Autodesk Inventor part; units mm, degrees
ref_plane "YZ Plane" through (0, 0, 0) normal (1, 0, 0) x (0, 1, 0)
ref_plane "XZ Plane" through (0, 0, 0) normal (0, 1, 0) x (-1, 0, 0)
ref_plane "XY Plane" through (0, 0, 0) normal (0, 0, 1) x (1, 0, 0)
sketch "Skizze1" plane through (0, 0, 0) normal (0, 0, 1) x (1, 0, 0)
  line L0 (-26, -30) -> (26, -30)
  line L1 (30, -26) -> (30, 26)
  line L2 (26, 30) -> (-26, 30)
  line L3 (-30, 26) -> (-30, -26)
  line L4 (-30, -30) -> (30, 30) construction
  line L5 (30, -30) -> (-30, 30) construction
  arc A0 (30, 26) -> (26, 30) centre (26, 26) ccw
  arc A1 (26, -30) -> (30, -26) centre (26, -26) ccw
  arc A2 (-30, -26) -> (-26, -30) centre (-26, -26) ccw
  arc A3 (-26, 30) -> (-30, 26) centre (-26, 26) ccw
  point P0 (0, 0)
  dimension "d0" = 4
  dimension "d1" = 60
extrude "Extrusion1" add sketch "Skizze1" against normal blind 100
sketch "Skizze2" plane through (0, 0, 0) normal (0, 0, 1) x (1, 0, 0)
  circle A0 centre (0, 0) radius 19.05
  dimension "d4" = 38.1
extrude "Extrusion2" add sketch "Skizze2" along normal blind 1.6
sketch "Skizze4" plane through (0, 0, 0) normal (0, 0, 1) x (1, 0, 0)
  circle A0 centre (0, 0) radius 19.05
  line L0 (30, 26) -> (30, -26)
  arc A1 (30, 26) -> (26, 30) centre (26, 26) ccw
  line L1 (-26, 30) -> (26, 30)
  arc A2 (-26, 30) -> (-30, 26) centre (-26, 26) ccw
  line L2 (-30, -26) -> (-30, 26)
  arc A3 (-30, -26) -> (-26, -30) centre (-26, -26) ccw
  line L3 (26, -30) -> (-26, -30)
  arc A4 (26, -30) -> (30, -26) centre (26, -26) ccw
  line L4 (26, -26) -> (-26, 26) construction
  line L5 (-23.57, 23.57) -> (23.57, 23.57) construction
  line L6 (23.57, 23.57) -> (23.57, -23.57) construction
  line L7 (23.57, -23.57) -> (-23.57, -23.57) construction
  line L8 (-23.57, -23.57) -> (-23.57, 23.57) construction
  line L9 (-23.57, 23.57) -> (23.57, -23.57) construction
  line L10 (23.57, 23.57) -> (-23.57, -23.57) construction
  dimension "d15" = 47.14
hole "Bohrung1" at (23.57, 23.57, 0) at (-23.57, 23.57, 0) at (-23.57, -23.57, 0) at (23.57, -23.57, 0) direction (0, 0, -1) diameter 4.5 end through all
sketch "Skizze5" plane through (0, 0, 1.6) normal (0, 0, 1) x (1, 0, 0)
  circle A0 centre (0, 0) radius 4
  dimension "d23" = 8
extrude "Extrusion4" add sketch "Skizze5" along normal blind 22.4
sketch "Skizze7" plane through (0, 0, -100) normal (0, 0, -1) x (-1, 0, 0)
  circle A0 centre (23.57, -23.57) radius 2.25
  circle A1 centre (-23.57, 23.57) radius 2.25
  circle A2 centre (23.57, 23.57) radius 2.25
  circle A3 centre (-23.57, -23.57) radius 2.25
  line L0 (-30, 26) -> (-30, -26)
  arc A4 (-30, -26) -> (-26, -30) centre (-26, -26) ccw
  line L1 (-26, -30) -> (26, -30)
  arc A5 (26, -30) -> (30, -26) centre (26, -26) ccw
  line L2 (30, -26) -> (30, 26)
  arc A6 (30, 26) -> (26, 30) centre (26, 26) ccw
  line L3 (26, 30) -> (-26, 30)
  arc A7 (-26, 30) -> (-30, 26) centre (-26, 26) ccw
  circle A8 centre (23.57, -23.57) radius 6.43 construction
  line L4 (30, -26) -> (30, 26)
  line L5 (30, -17.14) -> (23.57, -17.14)
  line L6 (-26, -30) -> (26, -30)
  line L7 (17.14, -30) -> (17.14, -23.57)
  arc A9 (23.57, -17.14) -> (17.14, -23.57) centre (23.57, -23.57) ccw
  arc A10 (-17.14, -23.57) -> (-23.57, -17.14) centre (-23.57, -23.57) ccw
  arc A11 (17.2019, 24.4599) -> (23.57, 17.14) centre (23.57, 23.57) ccw
  arc A12 (-23.57, 17.14) -> (-17.14, 23.57) centre (-23.57, 23.57) ccw
  line L8 (23.57, 17.14) -> (30, 17.14)
  line L9 (17.14, 23.57) -> (17.14, 30)
  line L10 (26, 30) -> (-26, 30)
  line L11 (-17.14, 23.57) -> (-17.14, 30)
  line L12 (-23.57, 17.14) -> (-30, 17.14)
  line L13 (-23.57, -17.14) -> (-30, -17.14)
  line L14 (-17.14, -23.57) -> (-17.14, -30)
  point P0 (0, 0)
extrude "Extrusion6" cut sketch "Skizze7" against normal blind 93.2 contours A7 L3 L11 A12 L12 L0 | L13 A10 L14 L1 A4 L0 | L3 A6 L2 L8 A11 L9 | L7 A9 L5 L2 A5 L1
sketch "Skizze8" plane through (0, 0, -100) normal (0, 0, -1) x (-1, 0, 0)
  circle A0 centre (23.57, -23.57) radius 2.25 construction
  circle A1 centre (-23.57, 23.57) radius 2.25 construction
  circle A2 centre (23.57, 23.57) radius 2.25 construction
  circle A3 centre (-23.57, -23.57) radius 2.25 construction
  circle A4 centre (0, 0) radius 19.05 construction
  line L0 (-30, 26) -> (-30, -26) construction
  arc A5 (-26, 30) -> (-30, 26) centre (-26, 26) ccw construction
  line L1 (26, 30) -> (-26, 30) construction
  arc A6 (30, 26) -> (26, 30) centre (26, 26) ccw construction
  line L2 (30, -26) -> (30, 26) construction
  arc A7 (26, -30) -> (30, -26) centre (26, -26) ccw construction
  line L3 (-26, -30) -> (26, -30) construction
  arc A8 (-30, -26) -> (-26, -30) centre (-26, -26) ccw construction
  circle A9 centre (0, 0) radius 42.4264 construction
  line L4 (30, 30) -> (-30, 30) construction
  line L5 (-30, 30) -> (-30, -30) construction
  line L6 (-30, -30) -> (30, -30) construction
  line L7 (30, -30) -> (30, 30) construction
  line L8 (30, 30) -> (-30, -30) construction
  line L9 (-30, 30) -> (30, -30) construction
  line L10 (-17.14, -30) -> (17.14, -30) construction
  line L11 (-30, 17.14) -> (-30, -17.14) construction
equation "\"d1\" = breite"
equation "\"d2\" = Laenge"
equation "\"d4\" = fit"
equation "\"d5\" = fit_l"
equation "\"d15\" = lochabstand"
equation "\"d16\" = bohrung_d"
equation "\"d23\" = schaft_d"
equation "\"d24\" = schaft_l"
equation "\"d28\" = Laenge - Mount_l"
equation "\"breite\" = 60"
equation "\"lochabstand\" = 47.14"
equation "\"schaft_d\" = 8"
equation "\"fit\" = 38.1"
equation "\"fit_l\" = 1.6"
equation "\"Mount_l\" = 6.8"
equation "\"Laenge\" = 100"
equation "\"bohrung_d\" = 4.5"
properties part number "Nema24 - L100" material "Stahl"
Work out the finished part from the listing and answer in its coordinate system (mm). A direction names the side the tool comes from. Coordinates: 2 decimals unless noted, no trailing zeros. Loops run counter-clockwise (first coordinate to the right, second up) from the corner with the lowest first, then second, coordinate; pieces in that order, holes last. Notation, with made-up numbers: M 23,-31.75 L 73,-31.75 A19 ccw 73,-15.75 Z; hole C -7,-7 d9. An arc over 180 degrees is marked long. Use CSV: the item, a comma, the result in double quotes. Start each with the question number.
(1) For faces 4 (the face through (27, 17.14, -54)), 5 (the face through (24, -26, -6.8)), 6 (the face through (-17.14, -27, -54)), 7 (the face through (-0.867, 3.905, 12.643)), determine the directions among +Z, -Z, +X, -X, +Y, -Y from which every point of the face is accessible in a straight line to the end or side of a thin tool.
(2) Find section A-A, the plane y = 0. Give the vertices of the cut face in (x, z).
(3) Find section C-C, the plane z = -40.5. Give the vertices of the cut face in (x, y), then the cut area to 3 significant figures.
(4) For a pull along X with two mould halves and no side action, classify faces 1 (the face through (-17.14, 27, -54)), 2 (the face through (-23, -26, -6.8)), 3 (the face through (25.566, 22.532, -3.448)) as +X half, -X half, draft (parallel to the pull), parting line (faces both ways), or undercut.
(5) Given pin 1 Ø6 at (x, y) = (-23.57, -23.57) entering from -Z; pin 2 Ø3 at (y, z) = (-27, -41.5) entering from -X; pin 3 Ø1.9 at (y, z) = (-28, -67) entering from +X; pin 4 Ø4 at (x, y) = (-23.57, 23.57) entering from -Z, each flat-ended and moving along its own axis, determine where each tip first touches the part or whether it passes through.
(6) Consider line 1 (Y direction, x = 23.57, z = -5.5); line 2 (X direction, y = 23, z = -4). Determine where each line is inside the solid, lowest interval first.
(7) Find section D-D, the plane x = 15.5. Give the vertices of the cut face in (y, z).
Recorded:
1,face 4,"-Z, +X, +Y"
1,face 5,"-Z, +X, -Y"
1,face 6,"-Z, -X, -Y"
1,face 7,"+Z"
2,outline,"M -30,-100 L 30,-100 L 30,0 L 19.05,0 L 19.05,1.6 L 4,1.6 L 4,24 L -4,24 L -4,1.6 L -19.05,1.6 L -19.05,0 L -30,0 Z"
3,outline,"M -30,-17.14 L -23.57,-17.14 A6.43 cw -17.14,-23.57 L -17.14,-30 L 17.14,-30 L 17.14,-23.57 A6.43 cw 23.57,-17.14 L 30,-17.14 L 30,17.14 L 23.57,17.14 A6.43 cw 17.14,23.57 L 17.14,30 L -17.14,30 L -17.14,23.57 A6.43 cw -23.57,17.14 L -30,17.14 Z"
3,area,"2,970 mm^2"
4,face 1,"-X half"
4,face 2,"draft"
4,face 3,"undercut"
5,pin 1,"stops at z = -6.8"
5,pin 2,"stops at x = -17.14"
5,pin 3,"stops at x = 17.14"
5,pin 4,"passes through"
6,line 1,"y = -30 to -25.82, -21.32 to 21.32, 25.82 to 30"
6,line 2,"x = -30 to -25.75, -21.39 to 21.39, 25.75 to 30"
7,outline,"M -30,-100 L 30,-100 L 30,0 L 11.07,0 L 11.07,1.6 L -11.07,1.6 L -11.07,0 L -30,0 Z"
